Autodesk Inventor part; units mm, degrees
ref_plane "YZ Plane" through (0, 0, 0) normal (1, 0, 0) x (0, 1, 0)
ref_plane "XZ Plane" through (0, 0, 0) normal (0, 1, 0) x (-1, 0, 0)
ref_plane "XY Plane" through (0, 0, 0) normal (0, 0, 1) x (1, 0, 0)
sketch "Skizze1" plane through (0, 0, 0) normal (0, 0, 1) x (1, 0, 0)
  line L0 (-22.6982, -31.5196) -> (-17.6982, -31.5196)
  line L1 (-17.6982, -31.5196) -> (-17.6982, -21.5196)
  line L2 (-17.6982, -21.5196) -> (25.3018, -21.5196)
  line L3 (25.3018, -21.5196) -> (25.3018, 21.4804)
  line L4 (25.3018, 21.4804) -> (-17.6982, 21.4804)
  line L5 (-17.6982, 21.4804) -> (-17.6982, 31.4804)
  line L6 (-17.6982, 31.4804) -> (-22.6982, 31.4804)
  line L7 (-22.6982, -31.5196) -> (-22.6982, 31.4804)
  point P0 (0, 0)
  dimension "d0" = 5
  dimension "d1" = 10
  dimension "d2" = 43
  dimension "d3" = 43
  dimension "d4" = 10
  dimension "d5" = 5
extrude "Extrusion1" add sketch "Skizze1" against normal blind 25
sketch "Skizze2" plane through (-22.6982, -31.5196, 0) normal (-1, 0, 0) x (0, 0, 1)
  line L0 (-25, 0) -> (-25, 63)
  line L1 (0, 63) -> (-25, 63)
  line L2 (-25, 0) -> (-20, 0)
  line L3 (-20, 0) -> (-20, 63)
  line L4 (-20, 63) -> (-25, 63)
  line L5 (-25, 63) -> (-25, 0)
  point P0 (0, 31.5196)
  dimension "d8" = 5
extrude "Extrusion2" add sketch "Skizze2" along normal blind 20
sketch "Skizze3" plane through (0, 0, -25) normal (0, 0, -1) x (-1, 0, 0)
  line L0 (12.9973, -21.5196) -> (-12.0027, -21.5196)
  line L1 (12.9973, -21.5196) -> (12.4967, 0.2869)
  line L2 (-12.0027, -21.5196) -> (-12.4994, 0.1188)
  arc A0 (12.4967, 0.2869) -> (-12.4994, 0.1188) centre (0, 0) ccw
  dimension "d12" = 25
extrude "Extrusion3" cut sketch "Skizze3" against normal blind 15
sketch "Skizze4" plane through (0, 0, -25) normal (0, 0, -1) x (-1, 0, 0)
  circle A0 centre (32.6982, -21.5196) radius 1.6
  line L0 (42.6982, 31.4804) -> (42.6982, -31.5196)
  line L1 (17.6982, -31.5196) -> (42.6982, -31.5196)
  circle A1 centre (32.6982, -1.5196) radius 1.6
  circle A2 centre (32.6982, 18.4804) radius 1.6
  point P0 (0, 0)
  dimension "d16" = 3.2
  dimension "d17" = 10
  dimension "d18" = 10
  dimension "d21" = 20
extrude "Extrusion4" cut sketch "Skizze4" against normal through all
fillet "Rundung1" radius 2 10 edges at (25.3018, -21.5196, -12.5) (-17.6982, -21.5196, -12.5) (25.3018, 21.4804, -12.5) (-17.6982, 21.4804, -12.5) (-17.6982, 31.4804, -12.5) (-17.6982, -31.5196, -12.5) (-42.6982, -31.5196, -22.5) (-42.6982, 31.4804, -22.5) (-12.9973, -21.5196, -17.5) (12.0027, -21.5196, -17.5)
sketch "Skizze5" plane through (0, 0, -25) normal (0, 0, -1) x (-1, 0, 0)
  circle A0 centre (15.5, -15.5) radius 1.6
  circle A1 centre (-15.5, -15.5) radius 1.6
  circle A2 centre (15.5, 15.5) radius 1.6
  circle A3 centre (-15.5, 15.5) radius 1.6
  point P0 (0, 0)
  dimension "d29" = 3.2
  dimension "d30" = 15.5
  dimension "d31" = 15.5
  dimension "d32" = 3.2
  dimension "d33" = 31
  dimension "d34" = 3.2
  dimension "d35" = 3.2
  dimension "d36" = 31
  dimension "d37" = 31
  dimension "d38" = 31
extrude "Extrusion5" cut sketch "Skizze5" against normal through all
sketch "Skizze6" plane through (-17.6982, 23.4804, 0) normal (1, 0, 0) x (0, 0, -1)
  circle A0 centre (10, 3) radius 1.6
  line L0 (0, 0) -> (0, 6)
  line L1 (25, 8) -> (0, 8)
  circle A1 centre (10, -50) radius 1.6
  line L2 (0, -55) -> (25, -55)
  line L3 (0, -53) -> (0, -47)
  point P0 (0, -23.4804)
  dimension "d41" = 3.2
  dimension "d42" = 10
  dimension "d43" = 5
  dimension "d44" = 3.2
  dimension "d45" = 5
  dimension "d46" = 10
extrude "Extrusion6" cut sketch "Skizze6" against normal through all
sketch "Skizze7" plane through (0, 0, 0) normal (0, 0, 1) x (1, 0, 0)
  circle A0 centre (15.5, -15.5) radius 1.6
  circle A1 centre (-15.5, -15.5) radius 1.6
  circle A2 centre (-15.5, 15.5) radius 1.6
  circle A3 centre (15.5, 15.5) radius 1.6
  circle A4 centre (15.5, -15.5) radius 3
  circle A5 centre (-15.5, -15.5) radius 3
  circle A6 centre (15.5, 15.5) radius 1.6
  circle A7 centre (15.5, 15.5) radius 3
  circle A8 centre (-15.5, 15.5) radius 3
  point P0 (0, 0)
  dimension "d49" = 6
  dimension "d50" = 6
  dimension "d51" = 6
  dimension "d52" = 6
extrude "Extrusion7" cut sketch "Skizze7" against normal blind 8
sketch "Skizze8" plane through (0, 0, -10) normal (0, 0, -1) x (-1, 0, 0)
  circle A0 centre (0, 0) radius 8.5
  dimension "d55" = 17
extrude "Extrusion8" cut sketch "Skizze8" against normal through all
chamfer "Fase1" distance 2 angle 45 2 edges at (8.5, 0, -10) (8.5, 0, 0)
properties part number "Y motor mount" material "ABS-Kunststoff"
Could you check a few things on this model? Use its own coordinates, in mm. A direction names the side the tool comes from. Coordinates: 2 decimals unless noted, no trailing zeros. Order: outer loops, then holes, each group sorted by start corner. A loop starts at its lowest first (then second) coordinate and runs counter-clockwise, first axis right, second up. Notation, with made-up numbers: (-23.75, -11.75) - (28.25, -11.75) arc R20 ccw to (28.25, -1.75) - close; hole circle Ø7 at (24.5, 26). An arc over 180 degrees is marked (long way). Answer in a Markdown table with one row per item. Add a question column.
(1) Will these pins go through, and if not, where does the flat tip stop? pin 1 (14.5 mm diameter, centred on x = 1, y = -12.5, fed in from -Z); pin 2 (7.5 mm diameter, centred on x = 13.5, z = -6.5, fed in from +Y); pin 3 (1.8 mm diameter, centred on x = -16.5, y = -14.5, fed in from +Z).
(2) If we section it at A-A, the plane y = 15.5: Please give me the cut outline in (x, z), then the cut area to 3 significant figures.
(3) If we section it at B-B, the plane x = 15.5: Please give me the cut outline in (y, z).
(4) On a 3-axis mill with a long thin cutter (end or side, diameter ignored), from which of +Z, -Z, +X, -X, +Y, -Y can I reach the whole of each face in a straight line? I mean faces 1 (the face through (-42.698, 0, -23)), 2 (the face through (-13.9, 15.57, -16.62)), 3 (the face through (-13.57, -20.965, -17.395)), 4 (the face through (-16.15, 12.57, -3.94)), 5 (the face through (4, 21.48, -12)). Say none if no direction works.
(5) If we section it at C-C, the plane z = -17.25: Please give me the cut outline in (x, y).
(6) I need wall thicknesses on L1, parallel to Y at x = 15.5, z = -14.25; L2, parallel to Y at x = 15.5, z = -3; L3, parallel to X at y = -25, z = -19.75. Which ranges of each line are inside material? Lowest first, please.
(7) If we mould it in two halves opening along Y, with no side actions, what happens to faces 6 (the face through (-17.698, 26, -12)), 7 (the face through (-42, 31, -23)), 8 (the face through (1.87, -8.42, -8.125))? For each: released by +Y, released by -Y, zero draft, split by the parting line, or undercut.
(8) If we section it at D-D, the plane z = -6: Please give me the cut outline in (x, y), then the cut area to 3 significant figures.
Results are:
| question | item | result |
|---|---|---|
| 1 | pin 1 | stops at z = -10 |
| 1 | pin 2 | stops at y = 21.48 |
| 1 | pin 3 | stops at z = -8 |
| 2 | outline | (-42.7, -25) - (-17.1, -25) - (-17.1, -8) - (-18.5, -8) - (-18.5, 0) - (-22.7, 0) - (-22.7, -20) - (-42.7, -20) - close; (-13.9, -25) - (13.9, -25) - (13.9, -8) - (12.5, -8) - (12.5, 0) - (-12.5, 0) - (-12.5, -8) - (-13.9, -8) - close; (17.1, -25) - (25.3, -25) - (25.3, 0) - (18.5, 0) - (18.5, -8) - (17.1, -8) - close |
| 2 | area | 1,100 mm2 |
| 3 | outline | (-21.52, -25) - (-17.1, -25) - (-17.1, -8) - (-18.5, -8) - (-18.5, 0) - (-21.52, 0) - close; (-13.9, -25) - (13.9, -25) - (13.9, -8) - (12.5, -8) - (12.5, 0) - (-12.5, 0) - (-12.5, -8) - (-13.9, -8) - close; (17.1, -25) - (21.48, -25) - (21.48, 0) - (18.5, 0) - (18.5, -8) - (17.1, -8) - close |
| 4 | face 1 | +Z, -Z, -X, +Y, -Y |
| 4 | face 2 | +Z, -Z |
| 4 | face 3 | -Z, -Y |
| 4 | face 4 | +Z |
| 4 | face 5 | +Z, -Z, +X, +Y |
| 5 | outline | (-22.7, -31.52) - (-19.7, -31.52) arc R2 ccw to (-17.7, -29.52) - (-17.7, -23.52) arc R2 cw to (-15.7, -21.52) - (-14.95, -21.52) arc R2 ccw to (-12.95, -19.57) - (-12.5, 0.29) arc R12.5 cw to (12.5, 0.12) - (12.05, -19.47) arc R2 ccw to (14.05, -21.52) - (23.3, -21.52) arc R2 ccw to (25.3, -19.52) - (25.3, 19.48) arc R2 ccw to (23.3, 21.48) - (-15.7, 21.48) arc R2 cw to (-17.7, 23.48) - (-17.7, 29.48) arc R2 ccw to (-19.7, 31.48) - (-22.7, 31.48) - close; hole circle Ø3.2 at (-15.5, -15.5); hole circle Ø3.2 at (-15.5, 15.5); hole circle Ø3.2 at (15.5, -15.5); hole circle Ø3.2 at (15.5, 15.5) |
| 6 | L1 | y = -21.52 to -17.1, -13.9 to 13.9, 17.1 to 21.48 |
| 6 | L2 | y = -21.52 to -18.5, -12.5 to 12.5, 18.5 to 21.48 |
| 6 | L3 | x = -22.7 to -17.7 |
| 7 | face 6 | zero draft |
| 7 | face 7 | released by +Y |
| 7 | face 8 | undercut |
| 8 | outline | (-22.7, -31.52) - (-19.7, -31.52) arc R2 ccw to (-17.7, -29.52) - (-17.7, -23.52) arc R2 cw to (-15.7, -21.52) - (23.3, -21.52) arc R2 ccw to (25.3, -19.52) - (25.3, 19.48) arc R2 ccw to (23.3, 21.48) - (-15.7, 21.48) arc R2 cw to (-17.7, 23.48) - (-17.7, 29.48) arc R2 ccw to (-19.7, 31.48) - (-22.7, 31.48) - close; hole circle Ø6 at (-15.5, -15.5); hole circle Ø6 at (-15.5, 15.5); hole circle Ø17 at (0, 0); hole circle Ø6 at (15.5, -15.5); hole circle Ø6 at (15.5, 15.5) |
| 8 | area | 1,820 mm2 |
